from build123d import *

# Parameters (mm, degrees)
F1_DEPTH = 20
F2_R     = 20
F4_DEPTH = 30


with BuildPart() as f1:
    # F0 (on Top) → F1 (new body)
    with BuildSketch(Plane.XY):
        Polygon((0, 100), (0, 0), (35, 0), (50, 50), (85, 50), (100, 65), (100, 100), align=None)
    extrude(amount=F1_DEPTH)

    # F2
    f2_edges = [f1.edges().sort_by_distance(p)[0] for p in [
        (50, 50, 10),
    ]]
    fillet(f2_edges, radius=F2_R)

    # F3 (on face) → F4 (join)
    with BuildSketch(Plane.XZ):
        with BuildLine():
            Line((35, 20), (35, 25))
            ThreePointArc((35, 25), (20, 40), (5, 25))
            Line((5, 25), (5, 20))
            Line((5, 20), (35, 20))
        make_face()
    extrude(amount=-F4_DEPTH)


solid = f1.part
Geometry check sheet. Reference: the model listing, model coordinates, mm. A direction names the side the tool comes from. Give positions to 0.01 mm unless a question says otherwise; leave off trailing zeros. Order: outer loops, then holes, each group sorted by start corner. A loop starts at its lowest first (then second) coordinate and runs counter-clockwise, first axis right, second up.
1. Sectioned sample at A-A (z = 5.5). Record the boundary of the cut face in (x, y).
Completed:
outline: (0, 0) - (35, 0) - (45.72, 35.75) arc R20 cw to (64.88, 50) - (85, 50) - (100, 65) - (100, 100) - (0, 100) - close
2. Access from +Z, -Z, +X, -X, +Y, -Y to the whole of each face (thin tool, end or side, straight path). Record for faces 1 (the face through (5, 15, 23)), 2 (the face through (75, 50, 10)), 3 (the face through (20, 30, 28)), 4 (the face through (35, 15, 22)).
Completed:
face 1: +Z, -X, +Y, -Y
face 2: +Z, -Z, +X, -Y
face 3: +Z, +X, -X, +Y
face 4: +Z, +X, +Y, -Y
3. Scan lines: line 1 (Y direction, x = 71, z = 10.5); line 2 (Z direction, x = 11.5, y = 81.5); line 3 (X direction, y = 19, z = 21.5). Record each from-to range of solid material in increasing order.
Completed:
line 1: y = 50 to 100
line 2: z = 0 to 20
line 3: x = 5 to 35
4. Sectioned sample at D-D (y = 51.5). Record the boundary of the cut face in (x, z).
Completed:
outline: (0, 0) - (86.5, 0) - (86.5, 20) - (0, 20) - close
5. Depth check by flat-ended pin: pin 1 (6 mm diameter, centred on x = 17, z = 33.5, fed in from +Y); pin 2 (12 mm diameter, centred on y = 56, z = 19.5, fed in from +X); pin 3 (16 mm diameter, centred on x = 73, z = 10, fed in from -Y); pin 4 (12 mm diameter, centred on y = 47.5, z = 29, fed in from +X). Enter the tip coordinate at first touch or a pass-through.
Completed:
pin 1: stops at y = 30
pin 2: stops at x = 97
pin 3: stops at y = 50
pin 4: passes through
6. Sectioned sample at B-B (x = 20). Record the boundary of the cut face in (y, z).
Completed:
outline: (0, 0) - (100, 0) - (100, 20) - (30, 20) - (30, 40) - (0, 40) - close
7. Sectioned sample at C-C (y = 27). Record the boundary of the cut face in (x, z).
Completed:
outline: (0, 0) - (43.1, 0) - (43.1, 20) - (35, 20) - (35, 25) arc R15 ccw to (5, 25) - (5, 20) - (0, 20) - close
